Read the model definition and answer for the solid it produces. Units are mm, in the model's axes. A direction names the side the tool comes from. Give positions to 0.01 mm unless a question says otherwise; leave off trailing zeros. Write each loop counter-clockwise with the first axis right and the second up, starting at its lowest first coordinate (ties: lowest second). Pieces come first, ordered by that corner, then holes. Notation, with made-up numbers: (27.5, -11.5) -> (51.5, -11.5) arc R5 cw to (51.5, -4.5) -> close; hole circle Ø10 at (-39.5, 34.25). An arc over 180 degrees is marked (long way). Answer as CSV lines item,"result". Start each with the question number.
1. A tool of negligible diameter and unlimited length cuts with its end or side. For faces 1 (the flat face through (49, 0, -7)), 2 (the cylindrical face through (99.859, -0.203, -7.395)), from which of +Z, -Z, +X, -X, +Y, -Y can it reach the whole face along a straight path? Write none if from no direction.
2. The part is cut by section D-D, the plane x = 94. Determine the outline of the cut face in (y, z), and give its area (3 significant figures).
3. For a pull along Z with two mould halves and no side action, classify faces 3 (the flat face through (100, -52, -7)), 4 (the cylindrical face through (100.62, -31.048, -11.066)) as pulls with the +Z half, pulls with the -Z half, needs draft (parallel to the pull), parting line crosses it, or undercut.
4. The part is cut by section C-C, the plane y = -16. Determine the outline of the cut face in (x, z), and give its area (3 significant figures).
5. The part is cut by section B-B, the plane x = 30. Determine the outline of the cut face in (y, z), and give its area (3 significant figures).
6. The part is cut by section A-A, the plane z = -11.5. Determine the outline of the cut face in (x, y), and give its area (3 significant figures).
7. Given pin 1 (3 mm diameter, centred on x = 53, z = -8, fed in from -Y); pin 2 (7.5 mm diameter, centred on y = -45.5, z = -10.5, fed in from -X), each flat-ended and moving along its own axis, determine where each tip first touches the part or whether it passes through.
8. Find the intervals of material crossed by line 1 (X direction, y = -94, z = -8.5); line 2 (Y direction, x = 77, z = -5.75); line 3 (X direction, y = 0.65, z = -11.5), in increasing order.
Autodesk Inventor part; units mm, degrees
ref_plane "YZ Plane" through (0, 0, 0) normal (1, 0, 0) x (0, 1, 0)
ref_plane "XZ Plane" through (0, 0, 0) normal (0, 1, 0) x (-1, 0, 0)
ref_plane "XY Plane" through (0, 0, 0) normal (0, 0, 1) x (1, 0, 0)
sketch "Sketch1" plane through (0, 0, 0) normal (0, 0, 1) x (1, 0, 0)
  line L0 (0, 0) -> (97, 0)
  line L1 (100, -3) -> (100, -100)
  arc A0 (100, -3) -> (97, 0) centre (97, -3) ccw
  point P0 (100, 0)
  dimension "d0" = 100
  dimension "d1" = 100
  dimension "d7" = 3
sketch "Sketch2" plane through (0, 0, 0) normal (1, 0, 0) x (0, 1, 0)
  line L0 (0, 0) -> (0, -15)
  line L1 (0, -15) -> (1, -15)
  line L2 (1, -15) -> (1, 0)
  line L3 (1, 0) -> (0, 0)
  dimension "d2" = 15
  dimension "d3" = 1
  dimension "d4" = 15
sweep "Sweep1" add profiles "Sketch2" path "Sketch1"
hole "Hole1" at (30, 1, -3.5) direction (0, -1, 0) diameter 4 end through all
hole "Hole2" at (67, 1, -11.5) direction (0, -1, 0) diameter 4 end through all
hole "Hole3" at (101, -33, -11.5) direction (-1, 0, 0) diameter 4 end through all
hole "Hole4" at (101, -70, -3.5) direction (-1, 0, 0) diameter 4 end through all
chamfer "Chamfer1" distance 0.25 angle 45 4 edges at (30, 0, -5.5) (67, 0, -13.5) (100, -33, -9.5) (100, -70, -1.5)
properties part number "80mmCornerBracket"
Results found:
1,face 1,"+Z, -Z, -X, -Y"
1,face 2,"+Z, -Z, +X, +Y"
2,outline,"(0, -15) -> (1, -15) -> (1, 0) -> (0, 0) -> close"
2,area,"15.0 mm²"
3,face 3,"needs draft"
3,face 4,"undercut"
4,outline,"(100, -15) -> (101, -15) -> (101, 0) -> (100, 0) -> close"
4,area,"15.0 mm²"
5,outline,"(0, -15) -> (1, -15) -> (1, -5.5) -> (0.25, -5.5) -> (0, -5.75) -> close; (0, -1.25) -> (0.25, -1.5) -> (1, -1.5) -> (1, 0) -> (0, 0) -> close"
5,area,"10.9 mm²"
6,outline,"(0, 0) -> (64.75, 0) -> (65, 0.25) -> (65, 1) -> (0, 1) -> close; (69, 0.25) -> (69.25, 0) -> (97, 0) arc R3 cw to (100, -3) -> (100, -30.75) -> (100.25, -31) -> (101, -31) -> (101, -3) arc R4 ccw to (97, 1) -> (69, 1) -> close; (100, -100) -> (101, -100) -> (101, -35) -> (100.25, -35) -> (100, -35.25) -> close"
6,area,"191 mm²"
7,pin 1,"stops at y = 0"
7,pin 2,"stops at x = 100"
8,line 1,"x = 100 to 101"
8,line 2,"y = 0 to 1"
8,line 3,"x = 0 to 65, 69 to 98.64"
